Source: CAD feature listing. Evaluate the final solid. Frame: model axes, mm. Face numbers are marked on the shaded views. Coordinates: 2 decimals unless noted, no trailing zeros. Order: outer loops, then holes, each group sorted by start corner. A loop starts at its lowest first (then second) coordinate and runs counter-clockwise, first axis right, second up.
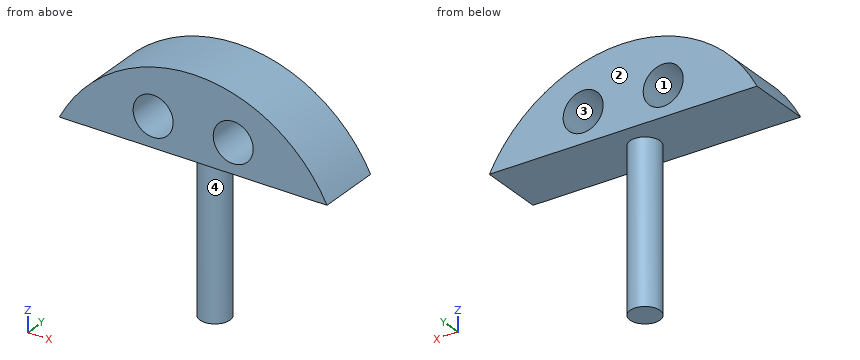
```python
from build123d import *

# Parameters (mm, degrees)
SKETCH1_R           = 6.35
BOSS_EXTRUDE1_DEPTH = 20.32
SKETCH2_R           = 4.7498
BOSS_EXTRUDE2_DEPTH = 50.8


with BuildPart() as part:
    # Sketch1 → Boss-Extrude1 (new body)
    with BuildSketch(Plane(origin=(0, 0, 0), x_dir=(1, 0, 0), z_dir=(0, 1, 0))):
        with BuildLine():
            Line((-42.460023894, -21.710352443), (42.460023894, -21.710352443))
            ThreePointArc((42.460023894, -21.710352443), (0, -47.6885), (-42.460023894, -21.710352443))
        make_face()
        with Locations(Location((-12.7, -31.235352443, 0), (0, 0, 270))):
            Circle(SKETCH1_R, mode=Mode.SUBTRACT)
        with Locations(Location((12.7, -31.235352443, 0), (0, 0, 270))):
            Circle(SKETCH1_R, mode=Mode.SUBTRACT)
    extrude(amount=BOSS_EXTRUDE1_DEPTH)

    # Sketch2 → Boss-Extrude2 (add)
    with BuildSketch(Plane(origin=(0, 0, 21.710352443), x_dir=(-1, 0, 0), z_dir=(0, 0, -1))):
        with Locations(Location((0, 10.16, 0), (0, 0, 180))):
            Circle(SKETCH2_R)
    extrude(amount=BOSS_EXTRUDE2_DEPTH)


solid = part.part
```
1. Section query D-D, the plane z = 27.5. Output: boundary loops of the cut face in (x, y).
2. Section query A-A, the plane y = 10.16. Output: boundary loops of the cut face in (x, z).
3. Draft query along X for the marked faces 1, 2, 3 and 4. Return one class per face: +X half, -X half, draft (parallel to the pull), parting line (faces both ways), or undercut.
4. Section query B-B, the plane x = 0. Output: boundary loops of the cut face in (y, z), plus the area to 3 significant figures.
5. Section query C-C, the plane x = -12.7. Output: boundary loops of the cut face in (y, z), plus the area to 3 significant figures.
6. Contact query for flat-ended pins moving along their axis: P1, Ø8, axis at x = 12, z = 39, coming from the -Y side; P2, Ø1.5, axis at x = -19, y = 5.5, coming from the +Z side; P3, Ø4, axis at x = -2, z = -4, coming from the +Y side; P4, Ø2, axis at x = -11, y = 4.5, coming from the +Z side. Output: stop coordinate, or through.
7. Material intervals for line 1 along X through (y, z) = (6.75, 32); line 2 along X through (y, z) = (3.25, 35); line 3 along Z through (x, y) = (-10, 9), sorted ascending.
Answer key:
1. outline: (-38.96, 0) - (-17.84, 0) - (-17.84, 20.32) - (-38.96, 20.32) - close; (-7.56, 0) - (7.56, 0) - (7.56, 20.32) - (-7.56, 20.32) - close; (17.84, 0) - (38.96, 0) - (38.96, 20.32) - (17.84, 20.32) - close
2. outline: (-42.46, 21.71) - (-4.75, 21.71) - (-4.75, -29.09) - (4.75, -29.09) - (4.75, 21.71) - (42.46, 21.71) arc R47.69 ccw to start; hole circle Ø12.7 at (-12.7, 31.24); hole circle Ø12.7 at (12.7, 31.24)
3. face 1: undercut
3. face 2: draft
3. face 3: undercut
3. face 4: parting line
4. outline: (0, 21.71) - (5.41, 21.71) - (5.41, -29.09) - (14.91, -29.09) - (14.91, 21.71) - (20.32, 21.71) - (20.32, 47.69) - (0, 47.69) - close
4. area: 1,010 mm2
5. outline: (0, 21.71) - (20.32, 21.71) - (20.32, 24.89) - (0, 24.89) - close; (0, 37.59) - (20.32, 37.59) - (20.32, 45.97) - (0, 45.97) - close
5. area: 235 mm2
6. P1: stops at y = 0
6. P2: stops at z = 44.06
6. P3: stops at y = 14.91
6. P4: stops at z = 46.63
7. line 1: x = -35.36 to -19, -6.4 to 6.4, 19 to 35.36
7. line 2: x = -32.39 to -17.81, -7.59 to 7.59, 17.81 to 32.39
7. line 3: z = 21.71 to 25.49, 36.98 to 46.63
